```python
from build123d import *

# Parameters (mm, degrees)
SKETCH_1_W      = 42
SKETCH_1_H      = 42
EXTRUDE_1_DEPTH = 40
SKETCH_1_3_R    = 11.5
EXTRUDE_2_DEPTH = 2
SKETCH_1_4_R    = 2.5
EXTRUDE_3_DEPTH = 16


with BuildPart() as part:
    # 草图1 → 凸台-拉伸1 (new body)
    with BuildSketch(Plane.XY):
        Rectangle(SKETCH_1_W, SKETCH_1_H)
    extrude(amount=EXTRUDE_1_DEPTH)

    # 草图1<3> → 凸台-拉伸2 (add)
    with BuildSketch(Plane.XY):
        Circle(SKETCH_1_3_R)
    extrude(amount=-EXTRUDE_2_DEPTH)

    # 草图1<4> → 凸台-拉伸3 (add)
    with BuildSketch(Plane.XY):
        Circle(SKETCH_1_4_R)
    extrude(amount=-EXTRUDE_3_DEPTH)

    # 草图2 → 旋转1 (revolve)
    with BuildSketch(Plane(origin=(0, 0, 0), x_dir=(1, 0, 0), z_dir=(0, 1, 0))):
        Polygon((2.5, 16), (7, 16), (7, 15), (6, 15), (6, 9), (7, 9), (7, 8), (2.5, 8), align=None)
    revolve(axis=Axis((0, 0, 1000), (0, 0, -1)))


solid = part.part
```
Here's how the part is built. I have some questions about the finished solid (model axes, mm). A direction names the side the tool comes from. Round coordinates to 2 decimals unless told otherwise and drop trailing zeros. Order: outer loops, then holes, each group sorted by start corner. A loop starts at its lowest first (then second) coordinate and runs counter-clockwise, first axis right, second up. Notation, with made-up numbers: (65.5, -21) -> (71.5, -21) arc R22 cw to (71.5, 6) -> close; hole circle Ø10 at (84.5, 56.5). An arc over 180 degrees is marked (long way). Use a Markdown table: item, result. Add a question column.
(1) I need wall thicknesses on line 1 along Z through (x, y) = (-2, 13.5); line 2 along Z through (x, y) = (-4, 7.5); line 3 along Z through (x, y) = (3, -0.5). Which ranges of each line are inside material? Lowest first, please.
(2) For pin 1 Ø1 at (y, z) = (0, -3.5) entering from +X; pin 2 Ø1.5 at (x, y) = (15, 17) entering from -Z, each with a flat end and sliding along its axis, tell me the tip position at first contact or that it passes through.
(3) Suppose I cut it at D-D, the plane x = 10.5. Please give me the cut outline in (y, z).
(4) Suppose I cut it at C-C, the plane x = -17. Please give me the cut outline in (y, z).
(5) Suppose I cut it at B-B, the plane x = 0. Please give me the cut outline in (y, z).
(6) If we mould it in two halves opening along Z, with no side actions, what happens to faces 1 (the face through (0, 0, 40)), 2 (the face through (-1.5, 11.4, -1)), 3 (the face through (-6, 0, -12))? For each: released by +Z, released by -Z, zero draft, split by the parting line, or undercut.
(7) For faces 4 (the face through (6, -2, -15)), 5 (the face through (-10, 10, 0)), 6 (the face through (21, 0, 20)), which set-ups out of +Z, -Z, +X, -X, +Y, -Y let a thin tool reach every point of the face, with its end or its side?
(8) Suppose I cut it at A-A, the plane x = -5. Please give me the cut outline in (y, z), and give its area (3 significant figures).
Verdict:
| question | item | result |
|---|---|---|
| 1 | line 1 | 0 to 40 |
| 1 | line 2 | -2 to 40 |
| 1 | line 3 | -16 to -8, -2 to 40 |
| 2 | pin 1 | x = 2.5 |
| 2 | pin 2 | z = 0 |
| 3 | outline | (-21, 0) -> (-4.69, 0) -> (-4.69, -2) -> (4.69, -2) -> (4.69, 0) -> (21, 0) -> (21, 40) -> (-21, 40) -> close |
| 4 | outline | (-21, 0) -> (21, 0) -> (21, 40) -> (-21, 40) -> close |
| 5 | outline | (-21, 0) -> (-11.5, 0) -> (-11.5, -2) -> (-2.5, -2) -> (-2.5, -8) -> (-7, -8) -> (-7, -9) -> (-6, -9) -> (-6, -15) -> (-7, -15) -> (-7, -16) -> (7, -16) -> (7, -15) -> (6, -15) -> (6, -9) -> (7, -9) -> (7, -8) -> (2.5, -8) -> (2.5, -2) -> (11.5, -2) -> (11.5, 0) -> (21, 0) -> (21, 40) -> (-21, 40) -> close |
| 6 | face 1 | released by +Z |
| 6 | face 2 | zero draft |
| 6 | face 3 | undercut |
| 7 | face 4 | none |
| 7 | face 5 | -Z |
| 7 | face 6 | +Z, -Z, +X, +Y, -Y |
| 8 | outline | (-21, 0) -> (-10.36, 0) -> (-10.36, -2) -> (10.36, -2) -> (10.36, 0) -> (21, 0) -> (21, 40) -> (-21, 40) -> close; (-4.9, -16) -> (4.9, -16) -> (4.9, -15) -> (3.32, -15) -> (3.32, -9) -> (4.9, -9) -> (4.9, -8) -> (-4.9, -8) -> (-4.9, -9) -> (-3.32, -9) -> (-3.32, -15) -> (-4.9, -15) -> close |
| 8 | area | 1,780 mm2 |
